Autodesk Inventor part; units mm, degrees
ref_plane "YZ Plane" through (0, 0, 0) normal (1, 0, 0) x (0, 1, 0)
ref_plane "XZ Plane" through (0, 0, 0) normal (0, 1, 0) x (-1, 0, 0)
ref_plane "XY Plane" through (0, 0, 0) normal (0, 0, 1) x (1, 0, 0)
sketch "Sketch1" plane through (0, 0, 0) normal (0, 0, 1) x (1, 0, 0)
  line L0 (2.3532, 14.024) -> (40.4532, 14.024)
  line L1 (40.4532, 14.024) -> (40.4532, -24.076)
  line L2 (40.4532, -24.076) -> (2.3532, -24.076)
  line L3 (2.3532, -24.076) -> (2.3532, 14.024)
  point P0 (0, 0)
  dimension "d0" = 38.1
  dimension "d1" = 38.1
extrude "Extrusion1" add sketch "Sketch1" along normal blind 38.1
sketch "Sketch2" plane through (0, 0, 38.1) normal (0, 0, 1) x (1, 0, 0)
  line L0 (15.0532, 14.024) -> (15.0532, 1.324)
  line L1 (40.4532, 14.024) -> (15.0532, 14.024)
  line L2 (15.0532, 14.024) -> (15.0532, -11.376)
  line L3 (15.0532, -11.376) -> (40.4532, -11.376)
  line L4 (40.4532, -11.376) -> (40.4532, 14.024)
  point P0 (0, 0)
  point P1 (2.3532, 14.024)
  point P2 (40.4532, -24.076)
  dimension "d5" = 12.7
extrude "Extrusion2" cut sketch "Sketch2" against normal through all
fillet "Fillet4" radius 3.175 1 edges at (15.0532, -11.376, 19.05)
chamfer "Chamfer5" distance 3.175 angle 45 1 edges at (15.0532, 14.024, 19.05)
chamfer "Chamfer6" distance 6.35 angle 45 1 edges at (40.4532, -11.376, 19.05)
properties part number "Chamfer Part"
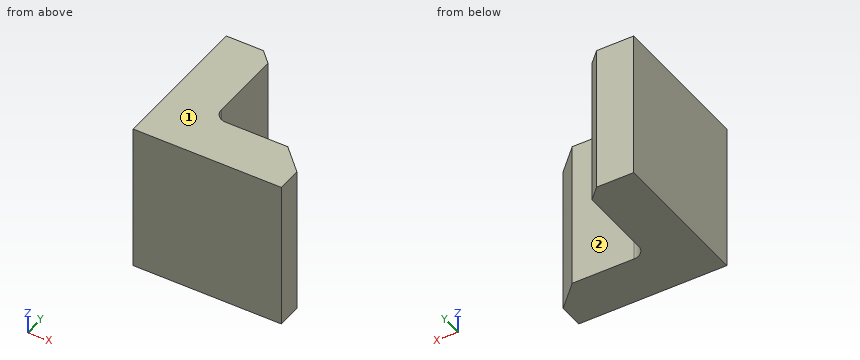
Source: CAD feature listing. Evaluate the final solid. Frame: model axes, mm. Face numbers are marked on the shaded views. A direction names the side the tool comes from. Coordinates: 2 decimals unless noted, no trailing zeros. Loops run counter-clockwise (first coordinate to the right, second up) from the corner with the lowest first, then second, coordinate; pieces in that order, holes last. Notation, with made-up numbers: (-32, 47.25) -> (-19, 47.25) arc R22 ccw to (-19, 76.25) -> close; hole circle Ø11 at (25, 44). An arc over 180 degrees is marked (long way). Answer in a Markdown table with one row per item. Add a question column.
Q1. Section C-C on x = 28. Return the cut outline in (y, z).
Q2. Contact query for flat-ended pins moving along their axis: pin 1 Ø8 at (x, z) = (29.5, 28) entering from +Y; pin 2 Ø2 at (y, z) = (9, 8) entering from +X. Output: stop coordinate, or through.
Q3. Reachability of the marked faces 1 and 2 from +Z, -Z, +X, -X, +Y, -Y: full face, straight path, thin tool, end or side. Return the list, or none.
Q4. Section A-A on z = 6.5. Return the cut outline in (x, y) (3 decimals), and give its area (3 significant figures).
Q5. Ray query, line 1 along Y through (x, z) = (27, 15.5); line 2 along X through (y, z) = (-4, 20); line 3 along X through (y, z) = (-11.5, 3.5). Return the intervals inside material, ascending.
Q6. Section B-B on y = 4. Return the cut outline in (x, z).
Computed values:
| question | item | result |
|---|---|---|
| 1 | outline | (-24.08, 0) -> (-11.38, 0) -> (-11.38, 38.1) -> (-24.08, 38.1) -> close |
| 2 | pin 1 | stops at y = -11.38 |
| 2 | pin 2 | stops at x = 15.05 |
| 3 | face 1 | +Z, +X, -X, +Y, -Y |
| 3 | face 2 | +Z, -Z, +X, +Y |
| 4 | outline | (2.353, -24.076) -> (40.453, -24.076) -> (40.453, -17.726) -> (34.103, -11.376) -> (18.228, -11.376) arc R3.175 cw to (15.053, -8.201) -> (15.053, 10.849) -> (11.878, 14.024) -> (2.353, 14.024) -> close |
| 4 | area | 783 mm^2 |
| 5 | line 1 | y = -24.08 to -11.38 |
| 5 | line 2 | x = 2.35 to 15.05 |
| 5 | line 3 | x = 2.35 to 34.23 |
| 6 | outline | (2.35, 0) -> (15.05, 0) -> (15.05, 38.1) -> (2.35, 38.1) -> close |
